from build123d import *

# Parameters (mm, degrees)
SKETCH1_W               = 41
SKETCH1_H               = 50
BOSS_EXTRUDE1_DEPTH     = 45
CUT_EXTRUDE1_DEPTH      = 59.85373316
CUT_EXTRUDE1_DEPTH_BACK = 10
SKETCH2_W               = 12
SKETCH2_H               = 10
CUT_EXTRUDE2_DEPTH      = 67.47818445
CUT_EXTRUDE2_DEPTH_BACK = 67.47818445
SKETCH3_R               = 8


with BuildPart() as part:
    # Sketch1 → Boss-Extrude1 (new body)
    with BuildSketch(Plane(origin=(0, 0, 0), x_dir=(1, 0, 0), z_dir=(0, 1, 0))):
        with Locations((6.433490288, 1.708594269)):
            Rectangle(SKETCH1_W, SKETCH1_H)
    extrude(amount=BOSS_EXTRUDE1_DEPTH)

    # Sketch2 → Cut-Extrude1 (cut, two sides: drawn at the far end of the back side and taken through both)
    with BuildSketch(Plane(origin=(0, 45, 0), x_dir=(1, 0, 0), z_dir=(0, 1, 0)).offset(-CUT_EXTRUDE1_DEPTH_BACK)):
        with Locations((-14.066509712, 1.708594269)):
            Rectangle(SKETCH2_W, SKETCH2_H)
    extrude(amount=CUT_EXTRUDE1_DEPTH + CUT_EXTRUDE1_DEPTH_BACK, mode=Mode.SUBTRACT)

    # Sketch3 → Cut-Extrude2 (cut, two sides: drawn at the far end of the back side and taken through both)
    with BuildSketch(Plane(origin=(26.933490288, 0, 0), x_dir=(0, 0, -1), z_dir=(1, 0, 0)).offset(-CUT_EXTRUDE2_DEPTH_BACK)):
        with Locations((0, -4.804588256)):
            Circle(SKETCH3_R)
    extrude(amount=CUT_EXTRUDE2_DEPTH + CUT_EXTRUDE2_DEPTH_BACK, mode=Mode.SUBTRACT)


solid = part.part
Source: CAD feature listing. Evaluate the final solid. Frame: model axes, mm. A direction names the side the tool comes from. Give positions to 0.01 mm unless a question says otherwise; leave off trailing zeros. Write each loop counter-clockwise with the first axis right and the second up, starting at its lowest first coordinate (ties: lowest second). Pieces come first, ordered by that corner, then holes. Notation, with made-up numbers: M 81.25,-18 L 135.25,-18 A19 cw 135.25,7 Z; hole C 41,1.25 d11. An arc over 180 degrees is marked long. Return JSON: item names as keys, results as strings. Group by question number.
1) Ray query, L1, parallel to Y at x = 14.5, z = -4; L2, parallel to Y at x = 14, z = 3. Return the intervals inside material, ascending.
2) Cut plane C-C, the plane z = -5.5. Output: boundary loops of the cut face in (x, y).
3) Cut plane A-A, the plane x = -9. Output: boundary loops of the cut face in (y, z), then the cut area to 3 significant figures.
4) Cut plane D-D, the plane z = -0.5. Output: boundary loops of the cut face in (x, y).
5) Set-up query: faces 4 (the face through (-11, 40, 3.291)), 5 (the face through (6, 0, -17)). Return all of +Z, -Z, +X, -X, +Y, -Y with unobstructed straight access to the full face (end or side cutting, diameter ignored); none if empty.
6) First-contact query: pin 1 Ø5 at (x, z) = (-6.5, 11) entering from -Y; pin 2 Ø3 at (x, z) = (5.5, 4) entering from -Y; pin 3 Ø5 at (x, z) = (-12.5, -1.5) entering from +Y. Flat tips, straight axial feed; report the tip coordinate or a pass-through.
7) Draft query along Z for faces 1 (the face through (-11, 35, -2)), 2 (the face through (-14.067, 22, -1)), 3 (the face through (6, 22, 23.291)). Return one class per face: released by +Z, released by -Z, zero draft, split by the parting line, or undercut.
8) Cut plane B-B, the plane y = 41.5. Output: boundary loops of the cut face in (x, z), then the cut area to 3 significant figures.
Data:
{
 "1": {"L1": "y = 2.12 to 45", "L2": "y = 2.61 to 45"},
 "2": {"outline": "M -14.07,1 L 26.93,1 L 26.93,45 L -8.07,45 L -8.07,35 L -14.07,35 Z"},
 "3": {"outline": "M 0,-26.71 L 45,-26.71 L 45,-6.71 L 35,-6.71 L 35,3.29 L 45,3.29 L 45,23.29 L 0,23.29 L 0,6.4 A8 cw 0,-6.4 Z", "area": "2,120 mm²"},
 "4": {"outline": "M -14.07,3.18 L 26.93,3.18 L 26.93,45 L -8.07,45 L -8.07,35 L -14.07,35 Z"},
 "5": {"face 4": "-X, +Y", "face 5": "+Z, -Z, +X, -X, -Y"},
 "6": {"pin 1": "stops at y = 0", "pin 2": "stops at y = 1", "pin 3": "stops at y = 35"},
 "7": {"face 1": "undercut", "face 2": "zero draft", "face 3": "released by +Z"},
 "8": {"outline": "M -14.07,-26.71 L 26.93,-26.71 L 26.93,23.29 L -14.07,23.29 L -14.07,3.29 L -8.07,3.29 L -8.07,-6.71 L -14.07,-6.71 Z", "area": "1,990 mm²"}
}
